```python
from build123d import *

# Parameters (mm, degrees)
SKETCH1_R           = 9.975
BOSS_EXTRUDE1_DEPTH = 3.15
FILLET1_R           = 0.5
CUT_EXTRUDE1_START  = -0.1
SKETCH3_R           = 9.3
SKETCH3_R_2         = 8.8
CUT_EXTRUDE1_DEPTH  = 0.1
FILLET2_R           = 0.3


with BuildPart() as part:
    # Sketch1 → Boss-Extrude1 (new body)
    with BuildSketch(Plane(origin=(0, 0, 0), x_dir=(1, 0, 0), z_dir=(0, 1, 0))):
        with Locations(Location((0, 0, 0), (0, 0, 270))):
            Circle(SKETCH1_R)
    extrude(amount=BOSS_EXTRUDE1_DEPTH)

    # Sketch2 → Cut-Revolve1 (revolve, cut)
    with BuildSketch(Plane.XY, mode=Mode.PRIVATE) as cut_revolve1_sk:
        with BuildLine():
            Line((8.8, 3.15), (8.8, 2.5))
            Line((8.8, 2.5), (9.3, 2.5))
            ThreePointArc((9.3, 2.5), (9.652003196, 2.448948287), (9.975, 2.3))
            Line((9.975, 2.3), (9.975, 3.15))
            Line((9.975, 3.15), (8.8, 3.15))
        make_face()
    revolve(cut_revolve1_sk.sketch.rotate(Axis((0, 0, 0), (0, 1, 0)), 90), axis=Axis((0, 0, 0), (0, 1, 0)), mode=Mode.SUBTRACT)

    # Fillet1
    fillet1_edges = [part.edges().sort_by_distance(p)[0] for p in [
        (0, 3.15, 8.8),
    ]]
    fillet(fillet1_edges, radius=FILLET1_R)

    # Sketch3 → Cut-Extrude1 (cut)
    with BuildSketch(Plane(origin=(0, 2.5, 0), x_dir=(1, 0, 0), z_dir=(0, 1, 0)).offset(CUT_EXTRUDE1_START)):
        with Locations(Location((0, 0, 0), (0, 0, 270))):
            Circle(SKETCH3_R)
        with Locations(Location((0, 0, 0), (0, 0, 270))):
            Circle(SKETCH3_R_2, mode=Mode.SUBTRACT)
    extrude(amount=CUT_EXTRUDE1_DEPTH, mode=Mode.SUBTRACT)

    # Fillet2
    fillet2_edges = [part.edges().sort_by_distance(p)[0] for p in [
        (0, 0, -9.975),
        (-9.975, 2.3, 0),
    ]]
    fillet(fillet2_edges, radius=FILLET2_R)


solid = part.part
```
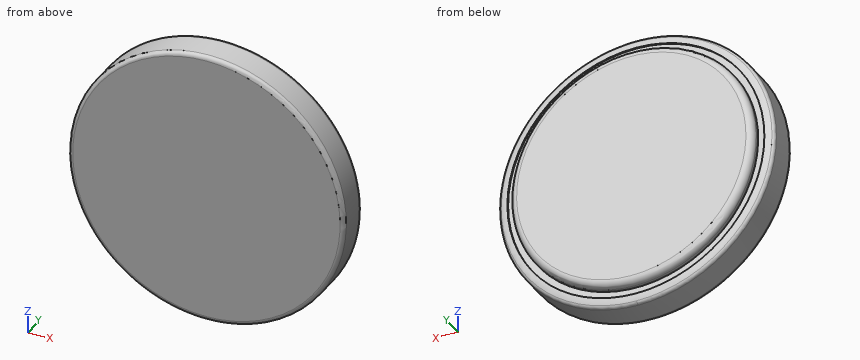
For this review, take the finished solid that the model builds, in its own axes (mm). Round coordinates to 2 decimals unless told otherwise and drop trailing zeros. Loops run counter-clockwise (first coordinate to the right, second up) from the corner with the lowest first, then second, coordinate; pieces in that order, holes last.
(1) Clearance check with a flat-ended pin moving along its axis: P1, Ø2, axis at x = -7.5, z = 5.5, coming from the -Y side. State where the tip first meets the part, or that it passes through.
Returned:
P1: stops at y = 0
(2) We need section A-A (y = 1). Give the boundary of the cut face in (x, z) (3 decimals), plus the area to 3 significant figures.
Returned:
outline: circle Ø19.95 at (0, 0)
area: 313 mm2
(3) Wall thickness on line 1 along Y through (x, z) = (-8, -4.25); line 2 along Y through (x, z) = (3.5, 9.25); line 3 along Z through (x, y) = (8.5, 0.2): over which ranges is each line inside the solid? List them lowest first.
Returned:
line 1: y = 0 to 2.4
line 2: y = 0.09 to 2.33
line 3: z = -5.19 to 5.19
